Geometry check sheet. Reference: drawing and pictorial views, mm from the part's lowest x, y, z. A direction names the side the tool comes from. Coordinates: 2 decimals unless noted, no trailing zeros. Loops run counter-clockwise (first coordinate to the right, second up) from the corner with the lowest first, then second, coordinate; pieces in that order, holes last. Notation, with made-up numbers: (1, 29) - (31, 29) arc R20 ccw to (31, 64) - close; hole circle Ø5 at (9.5, 77). An arc over 180 degrees is marked (long way). One line per item, written item: value.
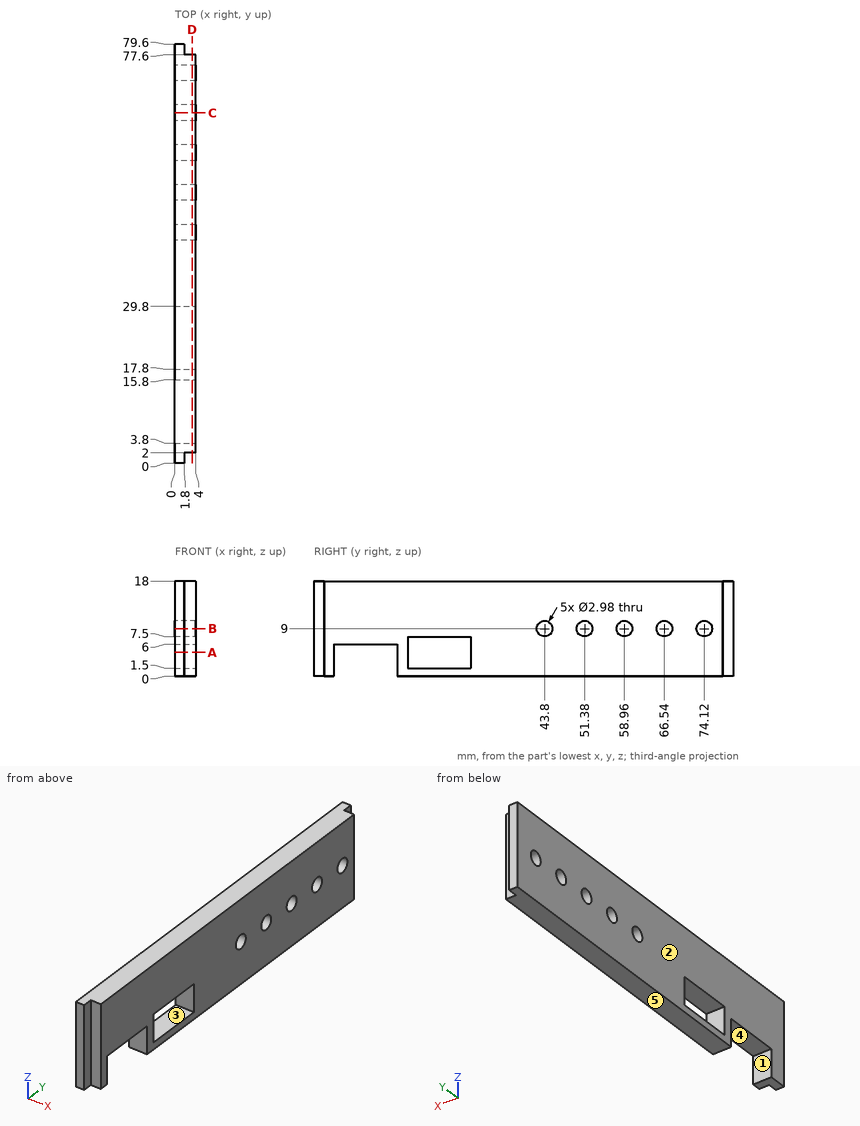
(1) Material ranges on probe 1 along Y at (x, z) = (1.9, 9); probe 2 along Y at (x, z) = (1.7, 9); probe 3 along Y at (x, z) = (2.5, 4), recorded low to high. Write a range as from..to.
Reply:
probe 1: 2..42.31, 45.29..49.89, 52.87..57.47, 60.45..65.05, 68.03..72.63, 75.61..77.6
probe 2: 0..42.31, 45.29..49.89, 52.87..57.47, 60.45..65.05, 68.03..72.63, 75.61..79.6
probe 3: 2..3.8, 15.8..17.8, 29.8..77.6
(2) Go/stop test with flat-tipped pins: pin 1 Ø1.6 at (y, z) = (78.5, 5.5) entering from +X; pin 2 Ø1.8 at (y, z) = (58.96, 9) entering from +X; pin 3 Ø0.7 at (x, z) = (2.5, 8) entering from +Y. Record where each tip stops, or that it passes through.
Reply:
pin 1: x = 1.8
pin 2: through
pin 3: y = 77.6
(3) Cross-section at C-C on y = 66.54. Record the cut outline in (x, z).
Reply:
outline: (0, 0) - (4, 0) - (4, 7.51) - (0, 7.51) - close; (0, 10.49) - (4, 10.49) - (4, 18) - (0, 18) - close
(4) Access from +Z, -Z, +X, -X, +Y, -Y to the whole of each face (thin tool, end or side, straight path). Record for the marked faces 1, 2 and 3.
Reply:
face 1: -Z, +X, -X
face 2: +Z, -Z, -X, +Y, -Y
face 3: +X, -X
(5) Cross-section at B-B on z = 9. Record the cut outline in (x, y), and give its area (3 significant figures).
Reply:
outline: (0, 0) - (1.8, 0) - (1.8, 2) - (4, 2) - (4, 42.31) - (0, 42.31) - close; (0, 45.29) - (4, 45.29) - (4, 49.89) - (0, 49.89) - close; (0, 52.87) - (4, 52.87) - (4, 57.47) - (0, 57.47) - close; (0, 60.45) - (4, 60.45) - (4, 65.05) - (0, 65.05) - close; (0, 68.03) - (4, 68.03) - (4, 72.63) - (0, 72.63) - close; (0, 75.61) - (4, 75.61) - (4, 77.6) - (1.8, 77.6) - (1.8, 79.6) - (0, 79.6) - close
area: 250 mm2
(6) Cross-section at D-D on x = 3.3. Record the cut outline in (y, z), and give its area (3 significant figures).
Reply:
outline: (2, 0) - (3.8, 0) - (3.8, 6) - (15.8, 6) - (15.8, 0) - (77.6, 0) - (77.6, 18) - (2, 18) - close; hole (17.8, 1.5) - (29.8, 1.5) - (29.8, 7.5) - (17.8, 7.5) - close; hole circle Ø2.98 at (43.8, 9); hole circle Ø2.98 at (51.38, 9); hole circle Ø2.98 at (58.96, 9); hole circle Ø2.98 at (66.54, 9); hole circle Ø2.98 at (74.12, 9)
area: 1,180 mm2
(7) Cross-section at A-A on z = 4.5. Record the cut outline in (x, y), and give its area (3 significant figures).
Reply:
outline: (0, 0) - (1.8, 0) - (1.8, 2) - (4, 2) - (4, 3.8) - (0, 3.8) - close; (0, 15.8) - (4, 15.8) - (4, 17.8) - (0, 17.8) - close; (0, 29.8) - (4, 29.8) - (4, 77.6) - (1.8, 77.6) - (1.8, 79.6) - (0, 79.6) - close
area: 214 mm2
(8) Release check for a two-part mould opening along Y. For the marked faces 4 and 5 record: pulls with the +Y half, pulls with the -Y half, needs draft (parallel to the pull), parting line crosses it, or undercut.
Reply:
face 4: undercut
face 5: needs draft
